```python
from build123d import *

# Parameters (mm, degrees)
SKETCH3_R          = 4.8125
CUT_EXTRUDE2_DEPTH = 51
CHAMFER1_SIZE      = 0.5


with BuildPart() as part:
    # Sketch1 → Revolve1 (revolve)
    with BuildSketch(Plane.XY):
        with BuildLine():
            Line((-25, 0), (25, 0))
            Line((25, 0), (25, -17))
            Line((25, -17), (14, -17))
            ThreePointArc((14, -17), (11, -14), (8, -17))
            Line((8, -17), (-8, -17))
            ThreePointArc((-8, -17), (-11, -14), (-14, -17))
            Line((-14, -17), (-25, -17))
            Line((-25, -17), (-25, 0))
        make_face()
    revolve(axis=Axis((-25, 0, 0), (1, 0, 0)))

    # Sketch3 → Cut-Extrude2 (cut, through all)
    with BuildSketch(Plane(origin=(25, 0, 0), x_dir=(0, 0, -1), z_dir=(1, 0, 0))):
        Circle(SKETCH3_R)
    extrude(amount=-CUT_EXTRUDE2_DEPTH, mode=Mode.SUBTRACT)

    # Chamfer1
    chamfer1_edges = [part.edges().sort_by_distance(p)[0] for p in [
        (25, 17, 0),
        (-25, 0, 4.8125),
        (25, 0, 4.8125),
        (-25, 17, 0),
    ]]
    chamfer(chamfer1_edges, length=CHAMFER1_SIZE)


solid = part.part
```
Check sheet for the modelled part. Datum: model origin and axes. Units: mm. Round coordinates to 2 decimals unless told otherwise and drop trailing zeros. Order: outer loops, then holes, each group sorted by start corner. A loop starts at its lowest first (then second) coordinate and runs counter-clockwise, first axis right, second up.
1) Scan lines: line 1 (X direction, y = 3.5, z = 14.5); line 2 (Y direction, x = 6, z = 0); line 3 (X direction, y = -11.5, z = 8.5). Record each from-to range of solid material in increasing order.
2) Section check D-D (z = 14.5). Give the number of separate pieces and of enclosed holes in the cut face, and give its area (3 significant figures).
3) Section check A-A (y = 0). Record the boundary of the cut face in (x, z), and give its area (3 significant figures).
4) Mould release check, pull along Z, two halves, no side actions. Record for faces 1 (the cylindrical face through (0.34, -2.93, 3.82)), 2 (the flat face through (25, -4, -4)), 3 (the cylindrical face through (19.176, -9.139, -14.334)): +Z half, -Z half, draft (parallel to the pull), parting line (faces both ways), or undercut.
5) Section check C-C (x = 5). Record the boundary of the cut face in (y, z) (1 decimal), and give its area (3 significant figures).
6) Go/stop test with flat-tipped pins: pin 1 Ø1.5 at (x, z) = (-3, 1.5) entering from -Y; pin 2 Ø12 at (x, y) = (18.5, -8) entering from -Z; pin 3 Ø6 at (x, z) = (9.5, 7) entering from +Y. Record where each tip stops, or that it passes through.
Result:
1. line 1: x = -25 to -13.16, -8.84 to 8.84, 13.16 to 25
1. line 2: y = -17 to -4.81, 4.81 to 17
1. line 3: x = -25 to -12.31, -9.69 to 9.69, 12.31 to 25
2. separate pieces: 3
2. enclosed holes: 0
2. area: 720 mm2
3. outline: (-25, -16.5) - (-24.5, -17) - (-14, -17) arc R3 cw to (-8, -17) - (8, -17) arc R3 cw to (14, -17) - (24.5, -17) - (25, -16.5) - (25, -5.31) - (24.5, -4.81) - (-24.5, -4.81) - (-25, -5.31) - close; (-25, 5.31) - (-24.5, 4.81) - (24.5, 4.81) - (25, 5.31) - (25, 16.5) - (24.5, 17) - (14, 17) arc R3 cw to (8, 17) - (-8, 17) arc R3 cw to (-14, 17) - (-24.5, 17) - (-25, 16.5) - close
3. area: 1,160 mm2
4. face 1: undercut
4. face 2: draft
4. face 3: parting line
5. outline: circle Ø34 at (0, 0); hole circle Ø9.6 at (0, 0)
5. area: 835 mm2
6. pin 1: stops at y = -16.98
6. pin 2: stops at z = -16.88
6. pin 3: stops at y = 16.42
